Geometry check sheet. Reference: drawing and pictorial views, mm from the part's lowest x, y, z. A direction names the side the tool comes from. Round coordinates to 2 decimals unless told otherwise and drop trailing zeros. Write each loop counter-clockwise with the first axis right and the second up, starting at its lowest first coordinate (ties: lowest second). Pieces come first, ordered by that corner, then holes. Notation, with made-up numbers: (40.25, 77) -> (47.25, 77) arc R33 cw to (47.25, 108) -> close; hole circle Ø1 at (66.5, -38). An arc over 180 degrees is marked (long way). Answer as a JSON object with one key per item and string values. Group by question number.
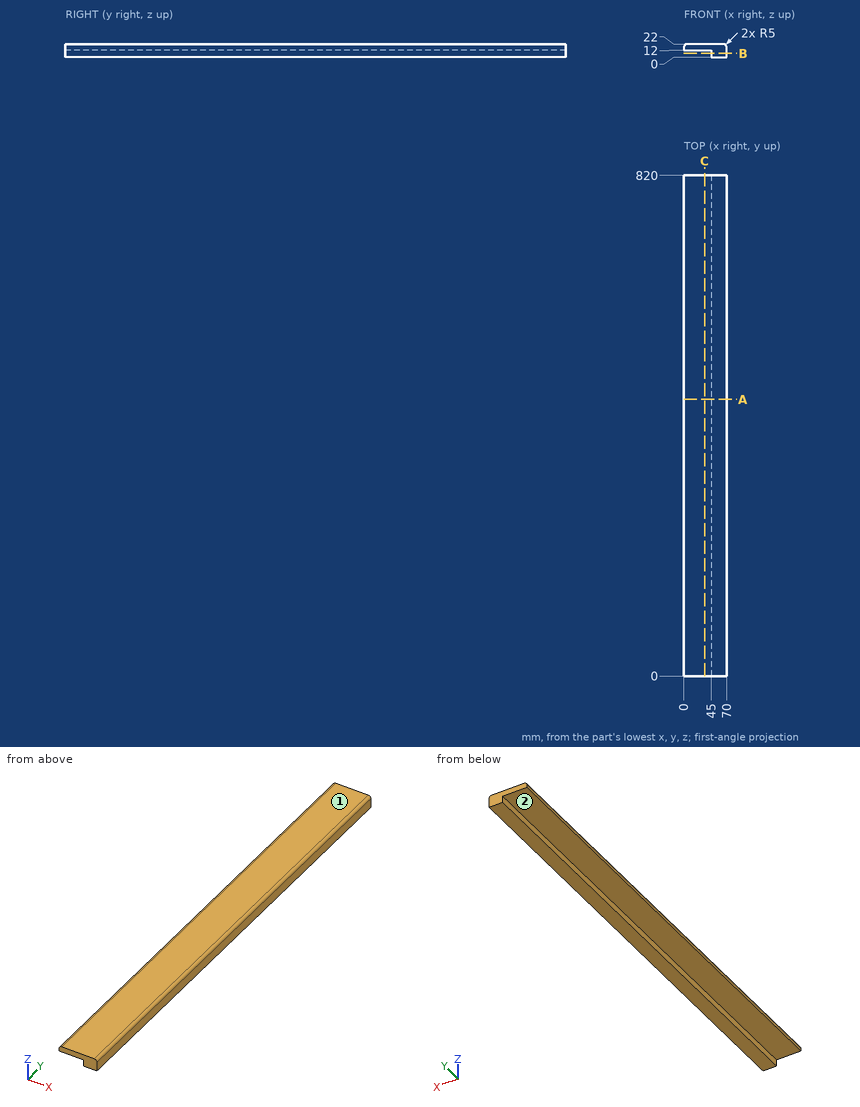
(1) Section check B-B on z = 6.75. Record the cut outline in (x, y).
(2) Go/stop test with flat-tipped pins: pin 1 Ø3.5 at (y, z) = (546, 6.5) entering from -X; pin 2 Ø1.5 at (y, z) = (353.5, 19.5) entering from -X; pin 3 Ø22.5 at (x, y) = (13.5, 273) entering from -Z. Record where each tip stops, or that it passes through.
(3) Access from +Z, -Z, +X, -X, +Y, -Y to the whole of each face (thin tool, end or side, straight path). Record for the marked faces 1 and 2.
(4) Section check A-A on y = 453. Record the cut outline in (x, z).
(5) Scan lines: line 1 along Z through (x, y) = (37.5, 783); line 2 along X through (y, z) = (146.5, 8); line 3 along X through (y, z) = (676.5, 18). Record each from-to range of solid material in increasing order.
(6) Section check C-C on x = 34. Record the cut outline in (y, z), then the cut area to 3 significant figures.
Data:
{
 "1": {"outline": "(45, 0) -> (70, 0) -> (70, 820) -> (45, 820) -> close"},
 "2": {"pin 1": "stops at x = 45", "pin 2": "stops at x = 0.32", "pin 3": "stops at z = 12"},
 "3": {"face 1": "+Z, +X, -X, +Y, -Y", "face 2": "-Z, -X, +Y, -Y"},
 "4": {"outline": "(0, 12) -> (45, 12) -> (45, 0) -> (70, 0) -> (70, 17) arc R5 ccw to (65, 22) -> (5, 22) arc R5 ccw to (0, 17) -> close"},
 "5": {"line 1": "z = 12 to 22", "line 2": "x = 45 to 70", "line 3": "x = 0.1 to 69.9"},
 "6": {"outline": "(0, 12) -> (820, 12) -> (820, 22) -> (0, 22) -> close", "area": "8,200 mm²"}
}
